Autodesk Inventor part; units mm, degrees
ref_plane "YZ Plane" through (0, 0, 0) normal (1, 0, 0) x (0, 1, 0)
ref_plane "XZ Plane" through (0, 0, 0) normal (0, 1, 0) x (-1, 0, 0)
ref_plane "XY Plane" through (0, 0, 0) normal (0, 0, 1) x (1, 0, 0)
sketch "Szkic1" plane through (0, 0, 0) normal (0, 1, 0) x (-1, 0, 0)
  line L0 (2, 0) -> (60, 0)
  line L1 (60, 0) -> (60, -18)
  line L2 (60, -18) -> (2, -18)
  line L3 (0, -16) -> (0, -2)
  circle A0 centre (9, -9) radius 2.5
  arc A1 (0, -16) -> (2, -18) centre (2, -16) ccw
  arc A2 (2, 0) -> (0, -2) centre (2, -2) ccw
  point P0 (0, 0)
  point P1 (0, -18)
  dimension "d0" = 60
  dimension "d1" = 18
  dimension "d2" = 5
  dimension "d3" = 9
  dimension "d4" = 9
  dimension "d5" = 2
extrude "Wyciągnięcie proste1" add sketch "Szkic1" along normal blind 1.6
equation "\"d4\" = 0.5 * d1"
properties part number "ramie3"
Design review of the part built by this model. Coordinates are the model's own, in mm. Round coordinates to 2 decimals unless told otherwise and drop trailing zeros. Write each loop counter-clockwise with the first axis right and the second up, starting at its lowest first coordinate (ties: lowest second). Pieces come first, ordered by that corner, then holes.
Item 1: Wall thickness on L1, parallel to Z at x = -9, y = 0.3; L2, parallel to Z at x = -10, y = 1.3; L3, parallel to X at y = 0.5, z = -10.25: over which ranges is each line inside the solid? List them lowest first.
Item 2: Consider section A-A on x = -9. Give the boundary of the cut face in (y, z).
Item 3: Consider section B-B on z = -9. Give the boundary of the cut face in (x, y), and give its area (3 significant figures).
Item 4: Consider section C-C on y = 1.05. Give the boundary of the cut face in (x, z), and give its area (3 significant figures).
Item 5: For pin 1 Ø4.5 at (x, z) = (-9, -9) entering from -Y, flat-tipped, find the tip position at first contact; note if it passes through.
Item 6: Draft analysis for pull direction X (two halves, no side actions). For faces 1 (the flat face through (-30, 1.6, -9)), 2 (the cylindrical face through (-8.46, 0.79, -6.56)), 3 (the cylindrical face through (-0.57, 0.79, -0.6)), state which applies: released by +X, released by -X, zero draft, split by the parting line, or undercut.
Check values:
1. L1: z = -18 to -11.5, -6.5 to 0
1. L2: z = -18 to -11.29, -6.71 to 0
1. L3: x = -60 to -11.17, -6.83 to 0
2. outline: (0, -18) - (1.6, -18) - (1.6, -11.5) - (0, -11.5) - close; (0, -6.5) - (1.6, -6.5) - (1.6, 0) - (0, 0) - close
3. outline: (-60, 0) - (-11.5, 0) - (-11.5, 1.6) - (-60, 1.6) - close; (-6.5, 0) - (0, 0) - (0, 1.6) - (-6.5, 1.6) - close
3. area: 88.0 mm2
4. outline: (-60, -18) - (-2, -18) arc R2 ccw to (0, -16) - (0, -2) arc R2 ccw to (-2, 0) - (-60, 0) - close; hole circle Ø5 at (-9, -9)
4. area: 1,060 mm2
5. pin 1: passes through
6. face 1: zero draft
6. face 2: undercut
6. face 3: released by +X
